```python
from build123d import *

# Parameters (mm, degrees)
SKETCH_1_R          = 40
SKETCH_1_R_2        = 24
EXTRUDE_1_DEPTH     = 1
SKETCH_2_R          = 2
CUT_EXTRUDE_1_DEPTH = 10
CUT_EXTRUDE_START   = -10
CUT_EXTRUDE_2_DEPTH = 10
FILLET_1_R          = 3


with BuildPart() as part:
    # 草图1 → 凸台-拉伸1 (new body)
    with BuildSketch(Plane.XY):
        Circle(SKETCH_1_R)
        Circle(SKETCH_1_R_2, mode=Mode.SUBTRACT)
    extrude(amount=EXTRUDE_1_DEPTH)

    # 草图2 → 切除-拉伸1 (cut)
    with BuildSketch(Plane.XY.offset(1)):
        with Locations((17.755280905, -21)):
            Circle(SKETCH_2_R)
        with Locations((17.755280905, 21)):
            Circle(SKETCH_2_R)
        with Locations((-17.755280905, -21)):
            Circle(SKETCH_2_R)
        with Locations((-17.755280905, 21)):
            Circle(SKETCH_2_R)
    extrude(amount=-CUT_EXTRUDE_1_DEPTH, mode=Mode.SUBTRACT)

    # 草图3 → 切除-拉伸2 (cut)
    with BuildSketch(Plane.XY.offset(1).offset(CUT_EXTRUDE_START)):
        with BuildLine():
            Line((12.616369605, -20.416346832), (16.558985107, -26.796455218))
            ThreePointArc((16.558985107, -26.796455218), (0, -31.5), (-16.558985107, -26.796455218))
            Line((-16.558985107, -26.796455218), (-12.616369605, -20.416346832))
            ThreePointArc((-12.616369605, -20.416346832), (0, -24), (12.616369605, -20.416346832))
        make_face()
        with BuildLine():
            Line((18.034256384, -15.835580086), (23.669961504, -20.784198863))
            ThreePointArc((23.669961504, -20.784198863), (31.5, 0), (23.669961504, 20.784198863))
            Line((23.669961504, 20.784198863), (18.034256384, 15.835580086))
            ThreePointArc((18.034256384, 15.835580086), (24, 0), (18.034256384, -15.835580086))
        make_face()
        with BuildLine():
            Line((12.616369605, 20.416346832), (16.558985107, 26.796455218))
            ThreePointArc((16.558985107, 26.796455218), (0, 31.5), (-16.558985107, 26.796455218))
            Line((-16.558985107, 26.796455218), (-12.616369605, 20.416346832))
            ThreePointArc((-12.616369605, 20.416346832), (0, 24), (12.616369605, 20.416346832))
        make_face()
        with BuildLine():
            Line((-18.034256384, 15.835580086), (-23.669961504, 20.784198863))
            ThreePointArc((-23.669961504, 20.784198863), (-31.5, 0), (-23.669961504, -20.784198863))
            Line((-23.669961504, -20.784198863), (-18.034256384, -15.835580086))
            ThreePointArc((-18.034256384, -15.835580086), (-24, 0), (-18.034256384, 15.835580086))
        make_face()
    extrude(amount=CUT_EXTRUDE_2_DEPTH, mode=Mode.SUBTRACT)

    # 圆角1
    fillet_1_edges = [part.edges().sort_by_distance(p)[0] for p in [
        (12.616369605, -20.416346832, 0.5),
        (-12.616369605, -20.416346832, 0.5),
        (18.034256384, 15.835580086, 0.5),
        (18.034256384, -15.835580086, 0.5),
        (12.616369605, 20.416346832, 0.5),
        (-12.616369605, 20.416346832, 0.5),
        (-18.034256384, 15.835580086, 0.5),
        (-18.034256384, -15.835580086, 0.5),
        (-23.669961504, -20.784198863, 0.5),
        (-23.669961504, 20.784198863, 0.5),
        (-16.558985107, 26.796455218, 0.5),
        (16.558985107, 26.796455218, 0.5),
        (23.669961504, 20.784198863, 0.5),
        (23.669961504, -20.784198863, 0.5),
        (16.558985107, -26.796455218, 0.5),
        (-16.558985107, -26.796455218, 0.5),
    ]]
    fillet(fillet_1_edges, radius=FILLET_1_R)


solid = part.part
```
The listing builds one solid part. Answer for the finished solid, in the listing's coordinates (mm). A direction names the side the tool comes from. Give positions to 0.01 mm unless a question says otherwise; leave off trailing zeros. Order: outer loops, then holes, each group sorted by start corner. A loop starts at its lowest first (then second) coordinate and runs counter-clockwise, first axis right, second up. Notation, with made-up numbers: (72, -39) -> (115, -39) arc R16 ccw to (115, -31) -> close; hole circle Ø4 at (14.5, 86). An arc over 180 degrees is marked (long way). Write each question's results on one line, items separated by ' | '.
Q1. The part is cut by section C-C, the plane y = -21. Give the vertices of the cut face in (x, z).
Checked values:
outline: (-34.04, 0) -> (-19.76, 0) -> (-19.76, 1) -> (-34.04, 1) -> close; (-15.76, 0) -> (-13.67, 0) -> (-13.67, 1) -> (-15.76, 1) -> close; (13.67, 0) -> (15.76, 0) -> (15.76, 1) -> (13.67, 1) -> close; (19.76, 0) -> (34.04, 0) -> (34.04, 1) -> (19.76, 1) -> close
Q2. The part is cut by section A-A, the plane y = 0. Give the vertices of the cut face in (x, z).
Checked values:
outline: (-40, 0) -> (-31.5, 0) -> (-31.5, 1) -> (-40, 1) -> close; (31.5, 0) -> (40, 0) -> (40, 1) -> (31.5, 1) -> close
Q3. Determine the mould class of faces 3 (the face through (16.28, 22.35, 0.51)), 4 (the face through (-18.3, -17.2, 1)), 5 (the face through (-8.67, -39.05, 0.49)) for opening direction Y: pulls with the +Y half, pulls with the -Y half, needs draft (parallel to the pull), parting line crosses it, or undercut.
Checked values:
face 3: undercut | face 4: needs draft | face 5: parting line crosses it
Q4. The part is cut by section D-D, the plane z = 0.3. State how many separate pieces and enclosed holes the cut face has, and give its area (3 significant figures).
Checked values:
separate pieces: 1 | enclosed holes: 5 | area: 2,110 mm^2
Q5. Straight lines are drawn through the part: probe 1 along Y at (x, z) = (-1, 0.25); probe 2 along Y at (x, z) = (18.5, 0.45); probe 3 along Y at (x, z) = (24, 0.9). For each, find the intervals that lie inside material, in ascending order. Write a range as from..to.
Checked values:
probe 1: y = -39.99..-31.48, 31.48..39.99 | probe 2: y = -35.46..-22.86, -19.14..-16.98, 16.98..19.14, 22.86..35.46 | probe 3: y = -32..-19.36, 19.36..32
Q6. Which of the six approach directions +Z, -Z, +X, -X, +Y, -Y give full straight-line access (tool end or side, diameter ignored) to faces 1 (the face through (0.2, 31.5, 0.5)), 2 (the face through (-18.3, -17.2, 0))?
Checked values:
face 1: +Z, -Z | face 2: -Z, +X, -X, +Y, -Y
